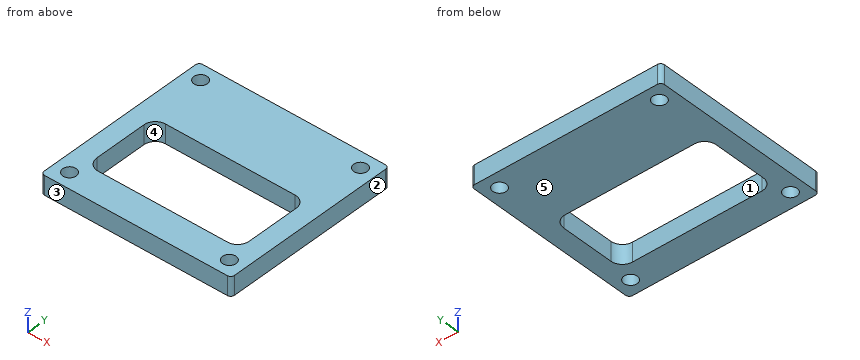
from build123d import *

# Parameters (mm, degrees)
SKETCH1_W             = 63.5
SKETCH1_H             = 59.69
BOSS_EXTRUDE1_DEPTH   = 6.35
FILLET1_R             = 1.27
F_8_CLEARANCE_HOLE1_D = 4.4958
SKETCH7_W             = 50.8
SKETCH7_H             = 25.4
CUT_EXTRUDE1_DEPTH    = 7.35
FILLET2_R             = 3.81


with BuildPart() as part:
    # Sketch1 → Boss-Extrude1 (new body)
    with BuildSketch(Plane.XY):
        with Locations((31.75, 29.845)):
            Rectangle(SKETCH1_W, SKETCH1_H)
    extrude(amount=BOSS_EXTRUDE1_DEPTH)

    # Fillet1
    fillet1_edges = [part.edges().sort_by_distance(p)[0] for p in [
        (0, 59.69, 3.175),
        (63.5, 59.69, 3.175),
        (63.5, 0, 3.175),
        (0, 0, 3.175),
    ]]
    fillet(fillet1_edges, radius=FILLET1_R)

    # #8 Clearance Hole1 (through all)
    with Locations(Plane.XY.offset(6.35)):
        with Locations((5.08, 54.61), (58.42, 54.61), (58.42, 5.08), (5.08, 5.08)):
            Hole(F_8_CLEARANCE_HOLE1_D / 2)

    # Sketch7 → Cut-Extrude1 (cut, through all)
    with BuildSketch(Plane.XY.offset(6.35)):
        with Locations((31.75, 22.86)):
            Rectangle(SKETCH7_W, SKETCH7_H)
    extrude(amount=-CUT_EXTRUDE1_DEPTH, mode=Mode.SUBTRACT)

    # Fillet2
    fillet2_edges = [part.edges().sort_by_distance(p)[0] for p in [
        (6.35, 10.16, 3.175),
        (6.35, 35.56, 3.175),
        (57.15, 35.56, 3.175),
        (57.15, 10.16, 3.175),
    ]]
    fillet(fillet2_edges, radius=FILLET2_R)


solid = part.part
Can you work these out from the model? Positions are in its coordinate system, mm. Face numbers are marked on the shaded views. A direction names the side the tool comes from. Give positions to 0.01 mm unless a question says otherwise; leave off trailing zeros. Order: outer loops, then holes, each group sorted by start corner. A loop starts at its lowest first (then second) coordinate and runs counter-clockwise, first axis right, second up. Notation, with made-up numbers: M 68,-3.75 L 75,-3.75 A31 cw 75,21.25 Z; hole C -37,-3.5 d11. An arc over 180 degrees is marked long. One line per item, written item: value.
Item 1: For the marked faces 4 and 5, which set-ups out of +Z, -Z, +X, -X, +Y, -Y let a thin tool reach every point of the face, with its end or its side?
Verdict:
face 4: +Z, -Z
face 5: -Z, +X, -X, +Y, -Y
Item 2: For pin 1 (3 mm diameter, centred on x = 42, y = 45, fed in from -Z), with a flat end and sliding along its axis, tell me the tip position at first contact or that it passes through.
Verdict:
pin 1: z = 0
Item 3: If we section it at B-B on x = 28: Write out the boundary of the cut face in (y, z), and give its area (3 significant figures).
Verdict:
outline: M 0,0 L 10.16,0 L 10.16,6.35 L 0,6.35 Z; M 35.56,0 L 59.69,0 L 59.69,6.35 L 35.56,6.35 Z
area: 218 mm2
Item 4: If we section it at C-C on y = 54.61: Write out the boundary of the cut face in (x, z).
Verdict:
outline: M 0,0 L 2.83,0 L 2.83,6.35 L 0,6.35 Z; M 7.33,0 L 56.17,0 L 56.17,6.35 L 7.33,6.35 Z; M 60.67,0 L 63.5,0 L 63.5,6.35 L 60.67,6.35 Z
Item 5: Please list where these lines run through material, in increasing order: line 1 (Y direction, x = 58.42, z = 2.75); line 2 (X direction, y = 27, z = 4.5); line 3 (Y direction, x = 39, z = 6).
Verdict:
line 1: 0 to 2.83, 7.33 to 52.36, 56.86 to 59.69
line 2: 0 to 6.35, 57.15 to 63.5
line 3: 0 to 10.16, 35.56 to 59.69
Item 6: If we section it at D-D on x = 58.42: Write out the boundary of the cut face in (y, z), and give its area (3 significant figures).
Verdict:
outline: M 0,0 L 2.83,0 L 2.83,6.35 L 0,6.35 Z; M 7.33,0 L 52.36,0 L 52.36,6.35 L 7.33,6.35 Z; M 56.86,0 L 59.69,0 L 59.69,6.35 L 56.86,6.35 Z
area: 322 mm2
Item 7: If we section it at A-A on y = 28: Write out the boundary of the cut face in (x, z).
Verdict:
outline: M 0,0 L 6.35,0 L 6.35,6.35 L 0,6.35 Z; M 57.15,0 L 63.5,0 L 63.5,6.35 L 57.15,6.35 Z
Item 8: If we mould it in two halves opening along X, with no side actions, what happens to the marked faces 1, 2 and 3? For each: pulls with the +X half, pulls with the -X half, needs draft (parallel to the pull), parting line crosses it, or undercut.
Verdict:
face 1: undercut
face 2: pulls with the +X half
face 3: needs draft
